from build123d import *

# Parameters (mm, degrees)
SKETCH1_R           = 0.6
BOSS_EXTRUDE1_DEPTH = 1.4
SKETCH2_R           = 3.5
BOSS_EXTRUDE2_DEPTH = 3.8
SKETCH3_R           = 2.3
CUT_EXTRUDE1_DEPTH  = 1
SKETCH4_R           = 2.5
CUT_EXTRUDE2_DEPTH  = 2
CUT_EXTRUDE3_REACH  = 18.908
SKETCH5_R           = 1.102182138


with BuildPart() as part:
    # Sketch1 → Boss-Extrude1 (new body)
    with BuildSketch(Plane(origin=(0, 0, 0), x_dir=(1, 0, 0), z_dir=(0, 1, 0))):
        with BuildLine():
            ThreePointArc((2.65, 2.286372673), (3.5, 0), (2.65, -2.286372673))
            Line((2.65, -2.286372673), (2, -14))
            ThreePointArc((2, -14), (0, -16), (-2, -14))
            Line((-2, -14), (-2.65, -2.286372673))
            ThreePointArc((-2.65, -2.286372673), (-3.5, 0), (-2.65, 2.286372673))
            Line((-2.65, 2.286372673), (-2, 14))
            ThreePointArc((-2, 14), (0, 16), (2, 14))
            Line((2, 14), (2.65, 2.286372673))
        make_face()
        with Locations(Location((0, -12.4, 0), (0, 0, 270))):
            Circle(SKETCH1_R, mode=Mode.SUBTRACT)
        with Locations(Location((0, -8.4, 0), (0, 0, 270))):
            Circle(SKETCH1_R, mode=Mode.SUBTRACT)
        with Locations(Location((0, -4.4, 0), (0, 0, 270))):
            Circle(SKETCH1_R, mode=Mode.SUBTRACT)
        with Locations(Location((0, 4.4, 0), (0, 0, 270))):
            Circle(SKETCH1_R, mode=Mode.SUBTRACT)
        with Locations(Location((0, 6.4, 0), (0, 0, 270))):
            Circle(SKETCH1_R, mode=Mode.SUBTRACT)
        with Locations(Location((0, 8.4, 0), (0, 0, 270))):
            Circle(SKETCH1_R, mode=Mode.SUBTRACT)
        with Locations(Location((0, 10.4, 0), (0, 0, 270))):
            Circle(SKETCH1_R, mode=Mode.SUBTRACT)
        with Locations(Location((0, 12.4, 0), (0, 0, 270))):
            Circle(SKETCH1_R, mode=Mode.SUBTRACT)
        with Locations(Location((0, 14.4, 0), (0, 0, 270))):
            Circle(SKETCH1_R, mode=Mode.SUBTRACT)
        with Locations(Location((0, -6.4, 0), (0, 0, 270))):
            Circle(SKETCH1_R, mode=Mode.SUBTRACT)
        with Locations(Location((0, -10.4, 0), (0, 0, 270))):
            Circle(SKETCH1_R, mode=Mode.SUBTRACT)
        with Locations(Location((0, -14.4, 0), (0, 0, 270))):
            Circle(SKETCH1_R, mode=Mode.SUBTRACT)
    extrude(amount=-BOSS_EXTRUDE1_DEPTH)

    # Sketch2 → Boss-Extrude2 (add)
    with BuildSketch(Plane(origin=(0, -1.4, 0), x_dir=(-1, 0, 0), z_dir=(0, -1, 0))):
        with Locations(Location((0, 0, 0), (0, 0, 319.212961807))):
            Circle(SKETCH2_R)
    extrude(amount=BOSS_EXTRUDE2_DEPTH)

    # Sketch3 → Cut-Extrude1 (cut)
    with BuildSketch(Plane(origin=(0, 0, 0), x_dir=(1, 0, 0), z_dir=(0, 1, 0))):
        with Locations(Location((0, 0, 0), (0, 0, 270))):
            Circle(SKETCH3_R)
    extrude(amount=-CUT_EXTRUDE1_DEPTH, mode=Mode.SUBTRACT)

    # Sketch4 → Cut-Extrude2 (cut)
    with BuildSketch(Plane(origin=(0, -5.2, 0), x_dir=(-1, 0, 0), z_dir=(0, -1, 0))):
        with Locations(Location((0, 0, 0), (0, 0, 90))):
            Circle(SKETCH4_R)
    extrude(amount=-CUT_EXTRUDE2_DEPTH, mode=Mode.SUBTRACT)

    # Sketch5 → Cut-Extrude3 (cut, up to next)
    with BuildSketch(Plane(origin=(0, -1, 0), x_dir=(1, 0, 0), z_dir=(0, 1, 0)), mode=Mode.PRIVATE) as cut_extrude3_sk1:
        with Locations(Location((0, 0, 0), (0, 0, 270))):
            Circle(SKETCH5_R)
    cut_extrude3_tool1 = extrude(cut_extrude3_sk1.sketch, amount=-CUT_EXTRUDE3_REACH, mode=Mode.PRIVATE) & part.part
    add(cut_extrude3_tool1.solids().sort_by_distance((0, -1, 0))[0], mode=Mode.SUBTRACT)


solid = part.part
Input: part model. Units: mm. Frame: model coordinates. A direction names the side the tool comes from. Coordinates: 2 decimals unless noted, no trailing zeros. Loops run counter-clockwise (first coordinate to the right, second up) from the corner with the lowest first, then second, coordinate; pieces in that order, holes last. Notation, with made-up numbers: (37, -32) - (87, -32) arc R17 ccw to (87, -1) - close; hole circle Ø6 at (51.5, 18.25). An arc over 180 degrees is marked (long way). Answer in a Markdown table with one row per item. Add a question column.
Item 1: Access query for faces 5 (the cylindrical face through (0.691, -0.493, 2.194)), 6 (the cylindrical face through (-2.44, -4.21, 0.54)), 7 (the cylindrical face through (1.093, -2.085, -0.143)). Directions: +Z, -Z, +X, -X, +Y, -Y. A direction counts if a zero-diameter tool reaches every point of the face in a straight line with its end or side. Return the directions, or none.
Item 2: Section query C-C on y = -2.25. Return the cut outline in (x, z).
Item 3: Line query: line 1 along X through (y, z) = (-1.9, 0); line 2 along X through (y, z) = (-3.75, 0); line 3 along Z through (x, y) = (-0.25, -4.1). Output: solid intervals per line, ascending. Write a range as [from, to].
Item 4: Section query B-B on x = 0. State how many separate pieces and enclosed holes the cut face has, then the cut area to 3 significant figures.
Item 5: Section query A-A on z = -12.4. Return the cut outline in (x, y), then the cut area to 3 significant figures.
Item 6: Section query D-D on x = 1.5. Return the cut outline in (y, z).
Item 7: Mould query, pull axis X, two halves, no side actions, for faces 1 (the flat face through (1, -1, 1)), 2 (the flat face through (0, -5.2, 3)), 3 (the flat face through (2.32, -0.69, -8.23)), 4 (the cylindrical face through (0, -1, -5)). Classes: released by +X, released by -X, zero draft, split by the parting line, or undercut.
Item 8: Contact query for flat-ended pins moving along their axis: P1, Ø1.1, axis at x = 0, z = 4.4, coming from the -Y side; P2, Ø1.6, axis at x = 0, z = -10.4, coming from the -Y side; P3, Ø1.5, axis at x = -1.5, y = -0.5, coming from the -Z side; P4, Ø3.5, axis at x = 0, z = 0, coming from the -Y side. Output: stop coordinate, or through.
Recorded:
| question | item | result |
|---|---|---|
| 1 | face 5 | +Y |
| 1 | face 6 | -Y |
| 1 | face 7 | +Y, -Y |
| 2 | outline | circle Ø7 at (0, 0); hole circle Ø2.2 at (0, 0) |
| 3 | line 1 | [-3.5, -1.1], [1.1, 3.5] |
| 3 | line 2 | [-3.5, -2.5], [2.5, 3.5] |
| 3 | line 3 | [-3.49, -2.49], [2.49, 3.49] |
| 4 | separate pieces | 14 |
| 4 | enclosed holes | 0 |
| 4 | area | 31.8 mm^2 |
| 5 | outline | (-2.09, -1.4) - (-0.6, -1.4) - (-0.6, 0) - (-2.09, 0) - close; (0.6, -1.4) - (2.09, -1.4) - (2.09, 0) - (0.6, 0) - close |
| 5 | area | 4.17 mm^2 |
| 6 | outline | (-5.2, -3.16) - (-1.4, -3.16) - (-1.4, -15.32) - (0, -15.32) - (0, -1.74) - (-1, -1.74) - (-1, 1.74) - (0, 1.74) - (0, 15.32) - (-1.4, 15.32) - (-1.4, 3.16) - (-5.2, 3.16) - (-5.2, 2) - (-3.2, 2) - (-3.2, -2) - (-5.2, -2) - close |
| 7 | face 1 | undercut |
| 7 | face 2 | zero draft |
| 7 | face 3 | released by +X |
| 7 | face 4 | undercut |
| 8 | P1 | through |
| 8 | P2 | y = -1.4 |
| 8 | P3 | z = -15.85 |
| 8 | P4 | y = -3.2 |
